```python
from build123d import *

# Parameters (mm, degrees)
SKETCH_1_W          = 40
SKETCH_1_H          = 24
SKETCH_1_R          = 2
EXTRUDE_1_DEPTH     = 3
SKETCH_2_W          = 20
SKETCH_2_H          = 6
EXTRUDE_2_DEPTH     = 25
SKETCH_3_R          = 8
CUT_EXTRUDE_1_DEPTH = 10


with BuildPart() as part:
    # 草图1 → 凸台-拉伸1 (new body)
    with BuildSketch(Plane(origin=(0, 0, 0), x_dir=(1, 0, 0), z_dir=(0, 1, 0))):
        Rectangle(SKETCH_1_W, SKETCH_1_H)
        with Locations((-14.8, -7.5)):
            Circle(SKETCH_1_R, mode=Mode.SUBTRACT)
        with Locations((14.8, -7.5)):
            Circle(SKETCH_1_R, mode=Mode.SUBTRACT)
        with Locations((-14.8, 7.5)):
            Circle(SKETCH_1_R, mode=Mode.SUBTRACT)
        with Locations((14.8, 7.5)):
            Circle(SKETCH_1_R, mode=Mode.SUBTRACT)
    extrude(amount=EXTRUDE_1_DEPTH)

    # 草图2 → 凸台-拉伸2 (add)
    with BuildSketch(Plane(origin=(0, 3, 0), x_dir=(1, 0, 0), z_dir=(0, 1, 0))):
        Rectangle(SKETCH_2_W, SKETCH_2_H)
    extrude(amount=EXTRUDE_2_DEPTH)

    # 草图3 → 切除-拉伸1 (cut)
    with BuildSketch(Plane.XY.offset(3)):
        with Locations((0, 17)):
            Circle(SKETCH_3_R)
    extrude(amount=-CUT_EXTRUDE_1_DEPTH, mode=Mode.SUBTRACT)


solid = part.part
```
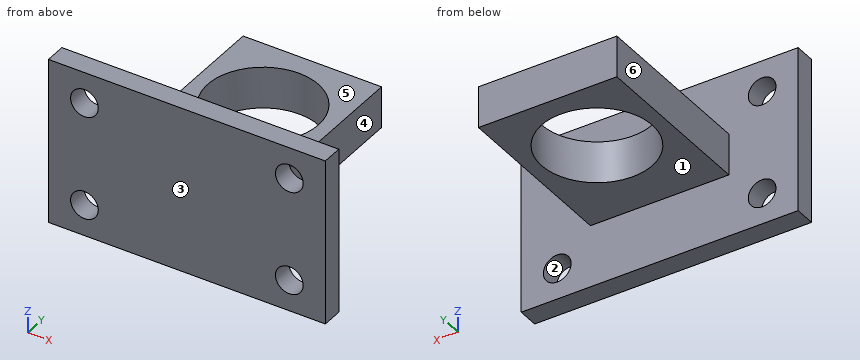
Input: part model. Units: mm. Frame: model coordinates. Face numbers are marked on the shaded views. A direction names the side the tool comes from. Coordinates: 2 decimals unless noted, no trailing zeros. Order: outer loops, then holes, each group sorted by start corner. A loop starts at its lowest first (then second) coordinate and runs counter-clockwise, first axis right, second up. Notation, with made-up numbers: (-27, 7.5) - (-17, 7.5) arc R29 ccw to (-17, 31.5) - close; hole circle Ø11 at (-18.75, 6.25). An arc over 180 degrees is marked (long way). Put each result on its own line as item: value.
1. Cut plane C-C on x = 14.8. Return the cut outline in (y, z).
Report:
outline: (0, -12) - (3, -12) - (3, -9.5) - (0, -9.5) - close; (0, -5.5) - (3, -5.5) - (3, 5.5) - (0, 5.5) - close; (0, 9.5) - (3, 9.5) - (3, 12) - (0, 12) - close
2. Draft query along Z for the marked faces 1, 2 and 3. Return one class per face: pulls with the +Z half, pulls with the -Z half, needs draft (parallel to the pull), parting line crosses it, or undercut.
Report:
face 1: pulls with the -Z half
face 2: undercut
face 3: needs draft
3. Cut plane D-D on x = -1.5. Return the cut outline in (y, z), then the cut area to 3 significant figures.
Report:
outline: (0, -12) - (3, -12) - (3, -3) - (9.14, -3) - (9.14, 3) - (3, 3) - (3, 12) - (0, 12) - close; (24.86, -3) - (28, -3) - (28, 3) - (24.86, 3) - close
area: 128 mm2
4. Cut plane B-B on z = 1.75. Return the cut outline in (x, y), then the cut area to 3 significant figures.
Report:
outline: (-20, 0) - (20, 0) - (20, 3) - (10, 3) - (10, 28) - (-10, 28) - (-10, 3) - (-20, 3) - close; hole circle Ø16 at (0, 17)
area: 419 mm2
5. Line query: line 1 along X through (y, z) = (1.25, 7.5); line 2 along Z through (x, y) = (14.8, 1.5); line 3 along Y through (x, z) = (0, 0.85). Output: solid intervals per line, ascending.
Report:
line 1: x = -20 to -16.8, -12.8 to 12.8, 16.8 to 20
line 2: z = -12 to -9.5, -5.5 to 5.5, 9.5 to 12
line 3: y = 0 to 9, 25 to 28
6. Cut plane A-A on y = 17. Return the cut outline in (x, z), then the cut area to 3 significant figures.
Report:
outline: (-10, -3) - (-8, -3) - (-8, 3) - (-10, 3) - close; (8, -3) - (10, -3) - (10, 3) - (8, 3) - close
area: 24.0 mm2
7. Contact query for flat-ended pins moving along their axis: pin 1 Ø10 at (x, y) = (-8.5, 20) entering from +Z; pin 2 Ø8 at (y, z) = (8, 4.5) entering from +X; pin 3 Ø5 at (x, z) = (-14.8, 7.5) entering from +Y; pin 4 Ø6 at (x, y) = (-1.5, 15) entering from +Z. Output: stop coordinate, or through.
Report:
pin 1: stops at z = 3
pin 2: stops at x = 10
pin 3: stops at y = 3
pin 4: passes through
8. Reachability of the marked faces 4, 5 and 6 from +Z, -Z, +X, -X, +Y, -Y: full face, straight path, thin tool, end or side. Return the list, or none.
Report:
face 4: +Z, -Z, +X, +Y
face 5: +Z, +X, -X, +Y
face 6: +Z, -Z, -X, +Y
